Can you work these out from the model? Positions are in its coordinate system, mm. A direction names the side the tool comes from. Round coordinates to 2 decimals unless told otherwise and drop trailing zeros. Order: outer loops, then holes, each group sorted by start corner. A loop starts at its lowest first (then second) coordinate and runs counter-clockwise, first axis right, second up. Notation, with made-up numbers: (10, 31.5) -> (57, 31.5) arc R33 ccw to (57, 70.5) -> close; hole circle Ø10 at (37.5, -23). An arc over 180 degrees is marked (long way). One line per item, written item: value.
Autodesk Fusion 360 part; units mm, degrees
sketch "Sketch1" plane through (0, 0, 0) normal (0, 1, 0) x (1, 0, 0)
  line L0 (-4.9858, 11.5) -> (-2.9364, 11.5)
  line L1 (8, 4.5467) -> (8, -8.4858)
  line L2 (4.9858, -11.5) -> (-4.9858, -11.5)
  line L3 (-8, -8.4858) -> (-8, 8.4858)
  line L4 (-8, 11.5) -> (8, -11.5) construction
  line L5 (8, 11.5) -> (-8, -11.5) construction
  circle A0 centre (-5.0352, 8.5) radius 1.325
  arc A1 (-0.3276, 9.9956) -> (4.6151, 7.538) centre (4, 12.5) ccw
  arc A2 (-4.9858, 11.5) -> (-8, 8.4858) centre (-4.9858, 8.4858) ccw
  arc A3 (-0.3276, 9.9956) -> (-2.9364, 11.5) centre (-2.9364, 8.4858) ccw
  arc A4 (8, 4.5467) -> (4.6151, 7.538) centre (4.9858, 4.5467) ccw
  arc A5 (4.9858, -11.5) -> (8, -8.4858) centre (4.9858, -8.4858) ccw
  arc A6 (-8, -8.4858) -> (-4.9858, -11.5) centre (-4.9858, -8.4858) ccw
  circle A7 centre (5, -8.5) radius 1.325
  dimension "d74" = 10
  dimension "d75" = 12
  dimension "d76" = 2.65
  dimension "d77" = 3
  dimension "d79" = 4
  dimension "d81" = 2.65
  dimension "d82" = 3
  dimension "d83" = 3
  dimension "d84" = 16
  dimension "d85" = 23
extrude "Extrude1" add sketch "Sketch1" against normal blind 2
ref_plane "WorkPlane1" through (0, 0, 2) normal (0, 0, 1) x (1, 0, 0)
sketch "Sketch14" plane through (0, 0, 2) normal (0, 0, 1) x (1, 0, 0)
  line L0 (-8, 0) -> (8, 0)
  circle A0 centre (0, 18) radius 2.5
  circle A1 centre (0, 27) radius 1.6
  arc A2 (8, 23) -> (0, 31) centre (0, 23) ccw
  line L1 (-8, 23) -> (-8, 0)
  arc A3 (0, 31) -> (-8, 23) centre (0, 23) ccw
  line L2 (8, 0) -> (8, 23)
  circle A4 centre (0, 9) radius 1.6
  point P0 (-8, 31)
  dimension "d64" = 16
  dimension "d65" = 31
  dimension "d66" = 3.2
  dimension "d67" = 3.2
  dimension "d68" = 18
  dimension "d69" = 5
  dimension "d70" = 9
  dimension "d71" = 8
extrude "Extrude8" add sketch "Sketch14" along normal mid plane 2
sketch "Sketch16" plane through (-8, 0, 0) normal (-1, 0, 0) x (0, 0, 1)
  line L0 (8.4858, 0) -> (3, 0)
  line L1 (3, 0) -> (3, 23)
  line L2 (3, 23) -> (1, 23)
  line L3 (1, 23) -> (1, 0)
  line L4 (1, 0) -> (-8.4858, 0)
  line L5 (-8.4858, 0) -> (-8.4858, -2)
  line L6 (-8.4858, -2) -> (8.4858, -2)
  line L7 (8.4858, -2) -> (8.4858, 0)
  line L8 (3, 23) -> (7.0555, 0)
  line L9 (3, 23) -> (26.3548, 23) construction
  dimension "d86" = 80
extrude "Extrude9" add sketch "Sketch16" against normal blind 2 contours L0 L1 L8
fillet "Fillet3" radius 2 1 edges at (1, 0, 3)
equation "d65 = 26 mm + 5 mm"
equation "d71 = ( 16 / 2 ) * 1 mm"
equation "d72 = ( 2 / 2 ) * 1 mm"
Q1. I want a section at A-A on y = 26. List the corners of the cut face in (x, z) for me.
Answers below:
outline: (-7.42, 1) -> (-1.25, 1) -> (-1.25, 3) -> (-7.42, 3) -> close; (1.25, 1) -> (7.42, 1) -> (7.42, 3) -> (1.25, 3) -> close
Q2. Will these pins go through, and if not, where does the flat tip stop? pin 1 Ø3 at (x, y) = (0, 9) entering from -Z; pin 2 Ø5 at (x, y) = (2, 19) entering from -Z; pin 3 Ø4 at (x, z) = (3.5, -7.5) entering from +Y; pin 4 Ø5 at (x, y) = (0, 27) entering from +Z.
Answers below:
pin 1: through
pin 2: z = 1
pin 3: y = 0
pin 4: z = 3
Q3. On a 3-axis mill with a long thin cutter (end or side, diameter ignored), from which of +Z, -Z, +X, -X, +Y, -Y can I reach the whole of each face in a straight line? I mean faces 1 (the face through (-6, 7, 4)), 2 (the face through (-7.14, -0.986, 10.594)), 3 (the face through (2, 16, 1)). Say none if no direction works.
Answers below:
face 1: +Z, +X, +Y
face 2: +Z, -X, +Y, -Y
face 3: -Z, +X, -X, +Y
Q4. I want a section at D-D on x = 7. List the corners of the cut face in (y, z) for me, plus the area to 3 significant figures.
Answers below:
outline: (-2, -6.79) -> (0, -6.79) -> (0, 1) -> (26.87, 1) -> (26.87, 3) -> (2, 3) arc R2 cw to (0, 5) -> (0, 10.73) -> (-2, 10.73) -> close
area: 89.6 mm^2
Q5. I want a section at B-B on x = -2. List the corners of the cut face in (y, z) for me.
Answers below:
outline: (-2, -11.35) -> (0, -11.35) -> (0, 1) -> (16.5, 1) -> (16.5, 3) -> (2, 3) arc R2 cw to (0, 5) -> (0, 11.5) -> (-2, 11.5) -> close; (19.5, 1) -> (30.75, 1) -> (30.75, 3) -> (19.5, 3) -> close
Q6. Please list where these lines run through material, in increasing order: line 1 along Y through (x, z) = (0, 2.5); line 2 along X through (y, z) = (-0.7, -8.5); line 3 along Z through (x, y) = (5, -1.3) (3 decimals).
Answers below:
line 1: -2 to 7.4, 10.6 to 15.5, 20.5 to 25.4, 28.6 to 31
line 2: -8 to -6.36, -3.71 to 1
line 3: -7.561 to 7.175, 9.825 to 11.5
Q7. I want a section at C-C on x = 0.75. List the corners of the cut face in (y, z) for me.
Answers below:
outline: (-2, -8.7) -> (0, -8.7) -> (0, 1) -> (7.59, 1) -> (7.59, 3) -> (2, 3) arc R2 cw to (0, 5) -> (0, 11.5) -> (-2, 11.5) -> close; (10.41, 1) -> (15.62, 1) -> (15.62, 3) -> (10.41, 3) -> close; (20.38, 1) -> (25.59, 1) -> (25.59, 3) -> (20.38, 3) -> close; (28.41, 1) -> (30.96, 1) -> (30.96, 3) -> (28.41, 3) -> close
Q8. We'd pull the mould along X, two halves only. Please class faces 4 (the face through (2.385, 17.249, 1.986)), 5 (the face through (-7.094, -0.986, -10.64)), 6 (the face through (-6.01, -0.99, -9.4)), 7 (the face through (7.094, -0.986, 10.64)): released by +X, released by -X, zero draft, split by the parting line, or undercut.
Answers below:
face 4: undercut
face 5: released by -X
face 6: undercut
face 7: released by +X
